The model under review builds one solid part; all positions refer to its coordinate system, in mm. A direction names the side the tool comes from. Coordinates: 2 decimals unless noted, no trailing zeros. Write each loop counter-clockwise with the first axis right and the second up, starting at its lowest first coordinate (ties: lowest second). Pieces come first, ordered by that corner, then holes. Notation, with made-up numbers: M 9.25,17 L 23.25,17 A22 cw 23.25,35 Z; hole C 34,81 d4. An arc over 180 degrees is marked long. Answer as a JSON object with one key per item and string values.
Autodesk Inventor part; units mm, degrees
ref_plane "YZ Plane" through (0, 0, 0) normal (1, 0, 0) x (0, 1, 0)
ref_plane "XZ Plane" through (0, 0, 0) normal (0, 1, 0) x (-1, 0, 0)
ref_plane "XY Plane" through (0, 0, 0) normal (0, 0, 1) x (1, 0, 0)
sketch "Sketch1" plane through (0, 0, 0) normal (0, 0, 1) x (1, 0, 0)
  line L0 (0, 0) -> (50.8, 0)
  line L1 (50.8, 0) -> (50.8, 20.066)
  line L2 (50.8, 20.066) -> (0, 20.066)
  line L3 (0, 20.066) -> (0, 0)
  line L4 (3.175, 20.066) -> (47.625, 20.066)
  line L5 (47.625, 20.066) -> (47.625, 23.241)
  line L6 (47.625, 23.241) -> (3.175, 23.241)
  line L7 (3.175, 23.241) -> (3.175, 20.066)
  line L8 (3.175, 0) -> (47.625, 0)
  line L9 (47.625, 0) -> (47.625, -3.175)
  line L10 (47.625, -3.175) -> (3.175, -3.175)
  line L11 (3.175, -3.175) -> (3.175, 0)
  point P0 (47.625, -1.5875)
  dimension "d0" = 3.175
  dimension "d1" = 3.175
  dimension "d2" = 3.175
  dimension "d3" = 3.175
  dimension "d4" = 3.175
  dimension "d5" = 3.175
  dimension "d6" = 44.45
  dimension "d7" = 20.066
extrude "Extrusion1" add sketch "Sketch1" along normal blind 3.175
properties part number "front support"
(1) For pin 1 Ø1.6 at (y, z) = (-2.5, 1.5) entering from +X (3 decimals); pin 2 Ø1.6 at (x, z) = (49, 2) entering from -Y; pin 3 Ø1.6 at (y, z) = (21.5, 2.5) entering from -X (3 decimals), all flat-tipped, find the tip position at first contact; note any pin that passes through.
Results list:
{"pin 1": "x = 47.625", "pin 2": "y = 0", "pin 3": "x = 3.175"}
(2) For faces 1 (the face through (49, 0, 2)), 2 (the face through (3.175, 22, 2)), 3 (the face through (2, 0, 2)), 4 (the face through (50.8, 10, 2)), 5 (the face through (49, 20.066, 2)), list the 3-axis set-ups (+Z, -Z, +X, -X, +Y, -Y) from which the entire face can be reached by the end or side of a thin tool; tool diameter is ignored.
Results list:
{"face 1": "+Z, -Z, +X, -Y", "face 2": "+Z, -Z, -X, +Y", "face 3": "+Z, -Z, -X, -Y", "face 4": "+Z, -Z, +X, +Y, -Y", "face 5": "+Z, -Z, +X, +Y"}
(3) Wall thickness on line 1 along Y through (x, z) = (48.5, 0.9); line 2 along X through (y, z) = (21.5, 2.95) (3 decimals): over which ranges is each line inside the solid? List them lowest first. Write a range as from..to.
Results list:
{"line 1": "0..20.07", "line 2": "3.175..47.625"}
(4) Add section A-A on z = 1.7. Give the boundary of the cut face in (x, y) (3 decimals), and give its area (3 significant figures).
Results list:
{"outline": "M 0,0 L 3.175,0 L 3.175,-3.175 L 47.625,-3.175 L 47.625,0 L 50.8,0 L 50.8,20.066 L 47.625,20.066 L 47.625,23.241 L 3.175,23.241 L 3.175,20.066 L 0,20.066 Z", "area": "1,300 mm²"}
